Can you work these out from the model? Positions are in its coordinate system, mm. A direction names the side the tool comes from. Give positions to 0.01 mm unless a question says otherwise; leave off trailing zeros. Write each loop counter-clockwise with the first axis right and the second up, starting at its lowest first coordinate (ties: lowest second). Pieces come first, ordered by that corner, then holes. Notation, with made-up numbers: (61, 28.5) -> (74, 28.5) arc R8 ccw to (74, 42.5) -> close; hole circle Ø1 at (75.25, 52.5). An arc over 180 degrees is marked (long way). One line per item, written item: value.
Autodesk Inventor part; units mm, degrees
ref_plane "YZ Plane" through (0, 0, 0) normal (1, 0, 0) x (0, 1, 0)
ref_plane "XZ Plane" through (0, 0, 0) normal (0, 1, 0) x (-1, 0, 0)
ref_plane "XY Plane" through (0, 0, 0) normal (0, 0, 1) x (1, 0, 0)
sketch "Эскиз1" plane through (0, 0, 0) normal (1, 0, 0) x (0, 1, 0)
  circle A0 centre (0, 0) radius 5
  circle A1 centre (0, -2.7) radius 0.6
  circle A2 centre (0, 0) radius 2.7 construction
  circle A3 centre (-2.3383, 1.35) radius 0.6
  circle A4 centre (2.3383, 1.35) radius 0.6
  line L0 (0, 0) -> (5.0108, 2.893) construction
  line L1 (0, 0) -> (-4.6178, 2.6661) construction
  line L2 (0, 0) -> (6.4667, 0) construction
  line L3 (0, 0) -> (-4.6765, -2.7) construction
  line L4 (0, 0) -> (4.6765, -2.7) construction
  circle A5 centre (-2.3383, -1.35) radius 0.6
  circle A6 centre (2.3383, -1.35) radius 0.6
  dimension "d1" = 10
  dimension "d3" = 1.2
  dimension "d24" = 5.4
  dimension "d25" = 1.2
  dimension "d26" = 1.2
  dimension "d53" = 120
  dimension "d54" = 30
  dimension "d55" = 120
  dimension "d56" = 30
  dimension "d57" = 1.2
  dimension "d58" = 1.2
extrude "Выдавливание1" add sketch "Эскиз1" along normal blind 6 contours A0 | A3 | A4 | A5 | A6
sketch "Эскиз6" plane through (6, 0, 0) normal (1, 0, 0) x (0, 0, -1)
  circle A0 centre (2.7, 0) radius 0.6
hole "Отверстие2" at (6, 0, -2.7) direction (-1, 0, 0) diameter 1.7 depth 3
extrude "Выдавливание2" cut sketch "Эскиз1" along normal blind 6 contours A3 | A4
sketch "Эскиз2" plane through (6, 0, 0) normal (1, 0, 0) x (0, 0, -1)
  point P0 (0, 0)
  point P1 (-1.35, 2.3383)
hole "Отверстие4" at (6, 2.3383, 1.35) direction (-1, 0, 0) diameter 1.7 depth 3
sketch "Эскиз3" plane through (6, 0, 0) normal (1, 0, 0) x (0, 0, -1)
  point P0 (0, 0)
  point P1 (-1.35, -2.3383)
hole "Отверстие5" at (6, -2.3383, 1.35) direction (-1, 0, 0) diameter 1.7 depth 3
extrude "Выдавливание3" cut sketch "Эскиз1" along normal blind 6 contours A5 | A6
sketch "Эскиз4" plane through (6, 0, 0) normal (1, 0, 0) x (0, 0, -1)
  point P0 (0, 0)
  point P1 (1.35, 2.3383)
hole "Отверстие6" at (6, 2.3383, -1.35) direction (-1, 0, 0) diameter 1.7 depth 3
sketch "Эскиз5" plane through (6, 0, 0) normal (1, 0, 0) x (0, 0, -1)
  point P0 (0, 0)
  point P1 (1.35, -2.3383)
hole "Отверстие7" at (6, -2.3383, -1.35) direction (-1, 0, 0) diameter 1.7 depth 3
equation "\"d1\" = inside"
equation "\"d3\" = 2 * pin_small_rad"
equation "\"d17\" = pin_big_dia"
properties part number "каркас" material "Пластмасса, непрозрачная, черная"
1) If we section it at D-D (z = -2.7): Write out the boundary of the cut face in (x, y), and give its area (3 significant figures).
Answer list:
outline: (0, -4.21) -> (6, -4.21) -> (6, -0.85) -> (3, -0.85) -> (3, -0.6) -> (0, -0.6) -> close; (0, 0.6) -> (3, 0.6) -> (3, 0.85) -> (6, 0.85) -> (6, 4.21) -> (0, 4.21) -> close
area: 41.8 mm^2
2) Will these pins go through, and if not, where does the flat tip stop? pin 1 (0.5 mm diameter, centred on y = 2, z = -1, fed in from +X); pin 2 (1 mm diameter, centred on x = 5, y = -2, fed in from -Z).
Answer list:
pin 1: stops at x = 3
pin 2: stops at z = -4.77
3) If we section it at B-B (z = 1.35): Write out the boundary of the cut face in (x, y).
Answer list:
outline: (0, -4.81) -> (6, -4.81) -> (6, -3.19) -> (3, -3.19) -> (3, -2.94) -> (0, -2.94) -> close; (0, -1.74) -> (3, -1.74) -> (3, -1.49) -> (6, -1.49) -> (6, 1.49) -> (3, 1.49) -> (3, 1.74) -> (0, 1.74) -> close; (0, 2.94) -> (3, 2.94) -> (3, 3.19) -> (6, 3.19) -> (6, 4.81) -> (0, 4.81) -> close
4) If we section it at A-A (y = 0): Write out the boundary of the cut face in (x, z), and give its area (3 significant figures).
Answer list:
outline: (0, -5) -> (6, -5) -> (6, -3.55) -> (3, -3.55) -> (3, -3.3) -> (0, -3.3) -> close; (0, -2.1) -> (3, -2.1) -> (3, -1.85) -> (6, -1.85) -> (6, 5) -> (0, 5) -> close
area: 51.3 mm^2
5) I need wall thicknesses on L1, parallel to Y at x = 2.1, z = -1.35; L2, parallel to Z at x = 5.7, y = 0; L3, parallel to Y at x = 5.6, z = -2. Which ranges of each line are inside material? Lowest first, please.
Answer list:
L1: y = -4.81 to -2.94, -1.74 to 1.74, 2.94 to 4.81
L2: z = -5 to -3.55, -1.85 to 5
L3: y = -4.58 to -2.89, -1.79 to -0.48, 0.48 to 1.79, 2.89 to 4.58
6) We'd pull the mould along Z, two halves only. Please class faces 1 (the face through (2.96, -1.08, 4.88)), 2 (the face through (4.48, 3.17, -1.17)), 3 (the face through (0, 0, 0)): released by +Z, released by -Z, zero draft, split by the parting line, or undercut.
Answer list:
face 1: split by the parting line
face 2: undercut
face 3: zero draft
7) If we section it at C-C (x = 1.45): Write out the boundary of the cut face in (y, z), and give its area (3 significant figures).
Answer list:
outline: circle Ø10 at (0, 0); hole circle Ø1.2 at (-2.34, -1.35); hole circle Ø1.2 at (-2.34, 1.35); hole circle Ø1.2 at (0, -2.7); hole circle Ø1.2 at (2.34, -1.35); hole circle Ø1.2 at (2.34, 1.35)
area: 72.9 mm^2
8) For faces 4 (the face through (4.48, 2.86, 2.02)), 5 (the face through (1.479, 1.862, 1.715)), which set-ups out of +Z, -Z, +X, -X, +Y, -Y let a thin tool reach every point of the face, with its end or its side?
Answer list:
face 4: +X
face 5: +X, -X
